```python
from build123d import *

# Parameters (mm, degrees)
SKETCH1_W           = 30
SKETCH1_H           = 20
BOSS_EXTRUDE1_DEPTH = 38
SKETCH2_W           = 12
SKETCH2_H           = 10
CUT_EXTRUDE1_DEPTH  = 38
SKETCH3_W           = 8
SKETCH3_H           = 8
CUT_EXTRUDE2_DEPTH  = 9
SKETCH4_W           = 2
SKETCH4_H           = 10
BOSS_EXTRUDE2_DEPTH = 12


with BuildPart() as part:
    # Sketch1 → Boss-Extrude1 (new body)
    with BuildSketch(Plane(origin=(0, 0, 0), x_dir=(1, 0, 0), z_dir=(0, 1, 0))):
        with Locations((15, 10)):
            Rectangle(SKETCH1_W, SKETCH1_H)
    extrude(amount=BOSS_EXTRUDE1_DEPTH)

    # Sketch2 → Cut-Extrude1 (cut)
    with BuildSketch(Plane.XY):
        with Locations((15, 19)):
            Rectangle(SKETCH2_W, SKETCH2_H)
    extrude(amount=-CUT_EXTRUDE1_DEPTH, mode=Mode.SUBTRACT)

    # Sketch3 → Cut-Extrude2 (cut)
    with BuildSketch(Plane(origin=(30, 0, 0), x_dir=(0, 0, -1), z_dir=(1, 0, 0))):
        with Locations((12, 19)):
            Rectangle(SKETCH3_W, SKETCH3_H)
    extrude(amount=-CUT_EXTRUDE2_DEPTH, mode=Mode.SUBTRACT)

    # Sketch4 → Boss-Extrude2 (add)
    with BuildSketch(Plane.ZY.offset(-21)):
        with Locations((-19, 19)):
            Rectangle(SKETCH4_W, SKETCH4_H)
    extrude(amount=BOSS_EXTRUDE2_DEPTH)


solid = part.part
```
Geometry: final body of the model. Coordinates: model frame, mm. A direction names the side the tool comes from. Coordinates: 2 decimals unless noted, no trailing zeros. Order: outer loops, then holes, each group sorted by start corner. A loop starts at its lowest first (then second) coordinate and runs counter-clockwise, first axis right, second up.
Item 1: Section query D-D (z = -14.5). Output: boundary loops of the cut face in (x, y).
Answer:
outline: (0, 0) - (30, 0) - (30, 15) - (21, 15) - (21, 14) - (9, 14) - (9, 24) - (21, 24) - (21, 23) - (30, 23) - (30, 38) - (0, 38) - close
Item 2: Section query C-C (y = 21). Output: boundary loops of the cut face in (x, z).
Answer:
outline: (0, -20) - (30, -20) - (30, -16) - (21, -16) - (21, -18) - (9, -18) - (9, 0) - (0, 0) - close; (21, -8) - (30, -8) - (30, 0) - (21, 0) - close
Item 3: Draft query along Y for faces 1 (the face through (15, 38, -10)), 2 (the face through (8, 19, 0)), 3 (the face through (26, 19, -8)). Return one class per face: released by +Y, released by -Y, zero draft, split by the parting line, or undercut.
Answer:
face 1: released by +Y
face 2: zero draft
face 3: undercut
Item 4: Section query A-A (x = 22.5). Output: boundary loops of the cut face in (y, z), then the cut area to 3 significant figures.
Answer:
outline: (0, -20) - (38, -20) - (38, 0) - (0, 0) - close; hole (15, -16) - (23, -16) - (23, -8) - (15, -8) - close
area: 696 mm2
Item 5: Section query B-B (z = -17.5). Output: boundary loops of the cut face in (x, y), then the cut area to 3 significant figures.
Answer:
outline: (0, 0) - (30, 0) - (30, 38) - (0, 38) - close; hole (9, 14) - (21, 14) - (21, 24) - (9, 24) - close
area: 1,020 mm2
Item 6: Contact query for a flat-ended pin moving along its axis: P1, Ø3, axis at x = 18, y = 17.5, coming from the +Z side. Output: stop coordinate, or through.
Answer:
P1: stops at z = -18
Item 7: Access query for faces 4 (the face through (26, 15, -12)), 5 (the face through (0, 19, -10)), 6 (the face through (15, 24, -9)). Directions: +Z, -Z, +X, -X, +Y, -Y. A direction counts if a zero-diameter tool reaches every point of the face in a straight line with its end or side. Return the directions, or none.
Answer:
face 4: +X
face 5: +Z, -Z, -X, +Y, -Y
face 6: +Z
Item 8: Material intervals for line 1 along Y through (x, z) = (28.25, -11); line 2 along Y through (x, z) = (10.25, -11); line 3 along X through (y, z) = (23, -0.75), sorted ascending.
Answer:
line 1: y = 0 to 15, 23 to 38
line 2: y = 0 to 14, 24 to 38
line 3: x = 0 to 9, 21 to 30
